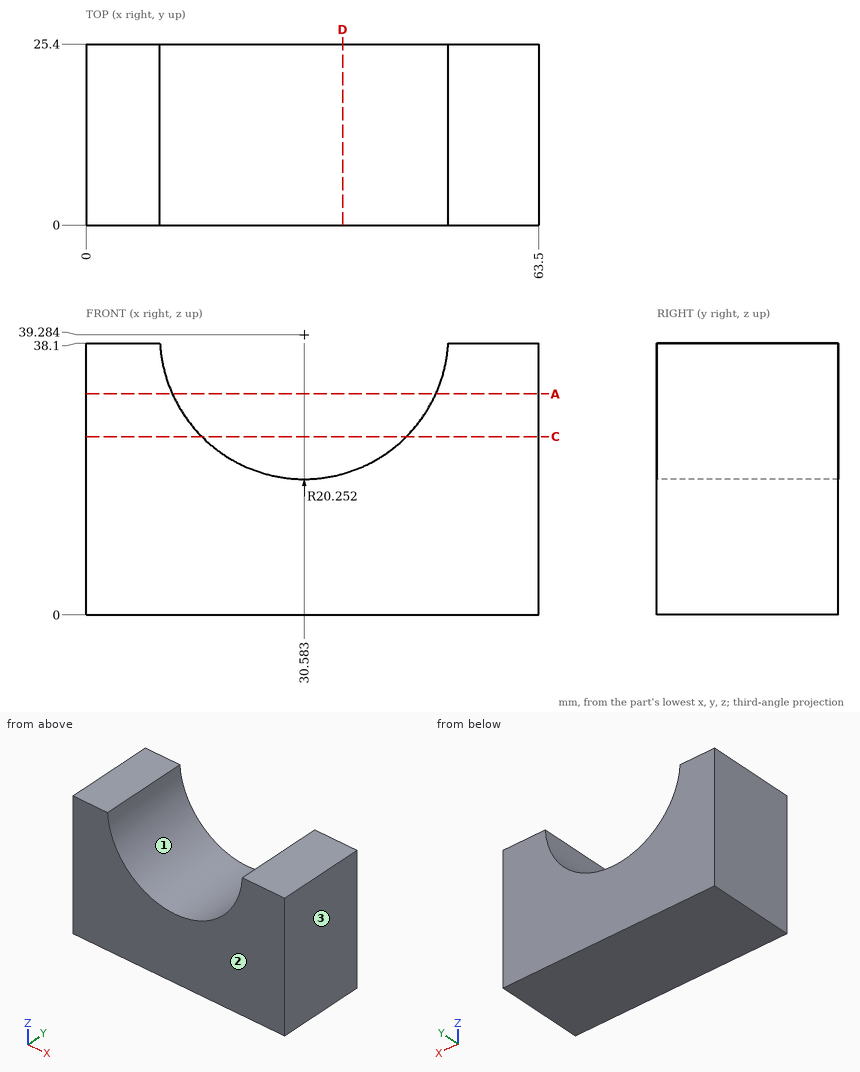
Geometry: see drawing. Coordinates: mm, zero at the bounding-box minimum. Coordinates: 2 decimals unless noted, no trailing zeros. Loops run counter-clockwise (first coordinate to the right, second up) from the corner with the lowest first, then second, coordinate; pieces in that order, holes last.
(1) Material intervals for probe 1 along X at (y, z) = (9.5, 25.5) (1 decimal); probe 2 along X at (y, z) = (22.75, 36.5); probe 3 along Z at (x, y) = (30, 21.5), sorted ascending.
(2) First-contact query: pin 1 Ø8 at (x, y) = (44, 21) entering from +Z; pin 2 Ø5 at (y, z) = (7.5, 20.5) entering from -X. Flat tips, straight axial feed; report the tip coordinate or a pass-through.
(3) Section A-A on z = 31. Return the cut outline in (x, y), then the cut area to 3 significant figures.
(4) Pull-direction query (X, two-part tool) for the marked faces 1, 2 and 3; classes: released by +X, released by -X, zero draft, split by the parting line, or undercut.
(5) Section C-C on z = 25. Return the cut outline in (x, y).
(6) Section D-D on x = 36. Return the cut outline in (y, z).
Data:
1. probe 1: x = 0 to 15.7, 45.4 to 63.5
1. probe 2: x = 0 to 10.52, 50.64 to 63.5
1. probe 3: z = 0 to 19.04
2. pin 1: stops at z = 28.95
2. pin 2: stops at x = 0
3. outline: (0, 0) - (12.1, 0) - (12.1, 25.4) - (0, 25.4) - close; (49.06, 0) - (63.5, 0) - (63.5, 25.4) - (49.06, 25.4) - close
3. area: 674 mm2
4. face 1: undercut
4. face 2: zero draft
4. face 3: released by +X
5. outline: (0, 0) - (16.23, 0) - (16.23, 25.4) - (0, 25.4) - close; (44.94, 0) - (63.5, 0) - (63.5, 25.4) - (44.94, 25.4) - close
6. outline: (0, 0) - (25.4, 0) - (25.4, 19.77) - (0, 19.77) - close
